The model under review builds one solid part; all positions refer to its coordinate system, in mm. Coordinates: 2 decimals unless noted, no trailing zeros. Write each loop counter-clockwise with the first axis right and the second up, starting at its lowest first coordinate (ties: lowest second). Pieces come first, ordered by that corner, then holes. Notation, with made-up numbers: (-28.75, 43.5) - (3.25, 43.5) arc R10 ccw to (3.25, 56.5) - close; hole circle Ø4 at (63.5, 27). An arc over 180 degrees is marked (long way). Put each result on its own line as item: value.
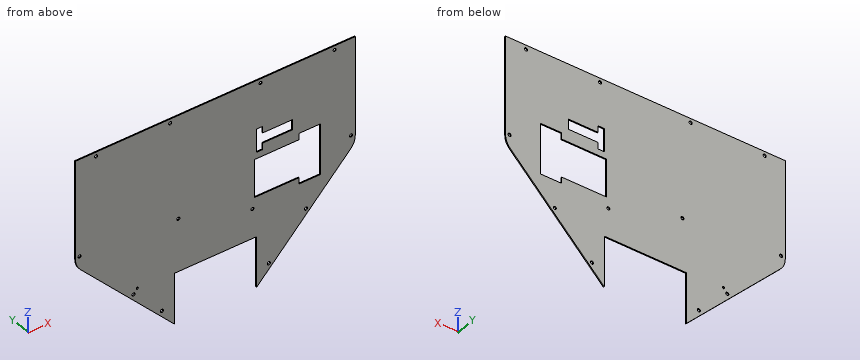
from build123d import *

# Parameters (mm, degrees)
EXTRUDE1_DEPTH     = 1.5875
MIRROR1_DEPTH      = 1.5875
CUT_EXTRUDE1_REACH = 534.229
SKETCH3_R          = 1.5875
CUT_EXTRUDE2_DEPTH = 533.229351555
SKETCH4_R          = 2.38125
SKETCH4_R_2        = 2.381250001
CUT_EXTRUDE3_DEPTH = 533.229351555
CUT_EXTRUDE4_DEPTH = 533.229351555
FILLET1_R          = 25.4


# Read off the part's stored shape, not the designer's step: Mirror1
with BuildPart() as part:
    # Sketch1 → Extrude1 (new body)
    with BuildSketch(Plane(origin=(0, 0, 0), x_dir=(1, 0, 0), z_dir=(0, 1, 0))):
        Polygon((0, 0), (0, 158.75), (152.4, 311.15), (152.4, 234.95), (215.9, 234.95), (215.9, 0), align=None)
    extrude(amount=EXTRUDE1_DEPTH)

    # Mirror1 outline → Mirror1 (add)
    with BuildSketch(Plane(origin=(0, 0, 0), x_dir=(1, 0, 0), z_dir=(0, 1, 0))):
        Polygon((215.9, 0), (431.8, 0), (431.8, 158.75), (279.4, 311.15), (279.4, 234.95), (215.9, 234.95), align=None)
    extrude(amount=MIRROR1_DEPTH)

    # Sketch2 → Cut-Extrude1 (cut, up to next)
    with BuildSketch(Plane(origin=(0, 1.5875, 0), x_dir=(-1, 0, 0), z_dir=(0, 1, 0)), mode=Mode.PRIVATE) as cut_extrude1_sk1:
        Polygon((-276.225, -174.625), (-345.059, -174.625), (-345.059, -184.15), (-377.825, -184.15), (-377.825, -107.95), (-345.059, -107.95), (-345.059, -117.475), (-276.225, -117.475), align=None)
    cut_extrude1_tool1 = extrude(cut_extrude1_sk1.sketch, amount=-CUT_EXTRUDE1_REACH, mode=Mode.PRIVATE) & part.part
    add(cut_extrude1_tool1.solids().sort_by_distance((330.365702, 1.5875, -146.05))[0], mode=Mode.SUBTRACT)

    # Sketch3 → Cut-Extrude2 (cut, through all)
    with BuildSketch(Plane.XZ):
        with Locations(Location((95.31871999, -232.5161053, 0), (0, 0, 270))):
            Circle(SKETCH3_R)
    extrude(amount=-CUT_EXTRUDE2_DEPTH, mode=Mode.SUBTRACT)

    # Sketch4 → Cut-Extrude3 (cut, through all)
    with BuildSketch(Plane.XZ):
        with Locations(Location((133.35, -283.119743879, 0), (0, 0, 270))):
            Circle(SKETCH4_R)
        with Locations(Location((273.05, -190.5, 0), (0, 0, 270))):
            Circle(SKETCH4_R)
        with Locations(Location((158.75, -155.575, 0), (0, 0, 270))):
            Circle(SKETCH4_R)
        with Locations(Location((298.45, -283.119743879, 0), (0, 0, 270))):
            Circle(SKETCH4_R)
        with Locations(Location((355.732177028, -225.837566851, 0), (0, 0, 270))):
            Circle(SKETCH4_R_2)
        with Locations(Location((425.45, -146.05, 0), (0, 0, 270))):
            Circle(SKETCH4_R)
        with Locations(Location((400.05, -6.35, 0), (0, 0, 270))):
            Circle(SKETCH4_R)
        with Locations(Location((31.75, -6.35, 0), (0, 0, 270))):
            Circle(SKETCH4_R)
        with Locations(Location((146.05, -6.35, 0), (0, 0, 270))):
            Circle(SKETCH4_R)
        with Locations(Location((285.75, -6.35, 0), (0, 0, 270))):
            Circle(SKETCH4_R)
        with Locations(Location((6.35, -146.05, 0), (0, 0, 270))):
            Circle(SKETCH4_R)
        with Locations(Location((89.563891484, -239.333635363, 0), (0, 0, 270))):
            Circle(SKETCH4_R)
    extrude(amount=-CUT_EXTRUDE3_DEPTH, mode=Mode.SUBTRACT)

    # Sketch5 → Cut-Extrude4 (cut, through all)
    with BuildSketch(Plane.XZ):
        Polygon((279.4, -107.9627), (279.4, -73.0123), (288.9504, -73.0123), (288.9504, -82.8675), (334.899, -82.8675), (334.899, -98.1075), (288.9504, -98.1075), (288.9504, -107.9627), align=None)
    extrude(amount=-CUT_EXTRUDE4_DEPTH, mode=Mode.SUBTRACT)

    # Fillet1
    fillet1_edges = [part.edges().sort_by_distance(p)[0] for p in [
        (0, 0.79375, -158.75),
        (431.8, 0.79375, -158.75),
    ]]
    fillet(fillet1_edges, radius=FILLET1_R)


solid = part.part
1. To check wall thickness, follow probe 1 along X at (y, z) = (0.85, -6.35); probe 2 along X at (y, z) = (0.2, -283); probe 3 along X at (y, z) = (1.3, -141.5) (3 decimals). State the ranges of each line that lie inside material, in increasing order.
Determined:
probe 1: x = 0 to 29.37, 34.13 to 143.67, 148.43 to 283.37, 288.13 to 397.67, 402.43 to 431.8
probe 2: x = 124.25 to 130.97, 135.73 to 152.4, 279.4 to 296.07, 300.83 to 307.55
probe 3: x = 0 to 276.225, 377.825 to 431.8
2. Consider section A-A on x = 324. Give the number of separate pieces and of enclosed holes in the cut face, plus the area to 3 significant figures.
Determined:
separate pieces: 3
enclosed holes: 0
area: 308 mm^2
3. For pin 1 Ø4.5 at (x, z) = (6.35, -146.05) entering from -Y; pin 2 Ø0.5 at (y, z) = (0.5, -180) entering from +X; pin 3 Ø0.8 at (y, z) = (0.5, -283.5) entering from -X, all flat-tipped, find the tip position at first contact; note any pin that passes through.
Determined:
pin 1: passes through
pin 2: stops at x = 410.8
pin 3: stops at x = 124.35
4. Consider section B-B on x = 123. State the section outline as (y, z) points, plus the area to 3 significant figures.
Determined:
outline: (0, -281.75) - (1.59, -281.75) - (1.59, 0) - (0, 0) - close
area: 447 mm^2
5. Consider section D-D on x = 185. State the section outline as (y, z) points.
Determined:
outline: (0, -234.95) - (1.59, -234.95) - (1.59, 0) - (0, 0) - close
